Geometry check sheet. Reference: the model listing, model coordinates, mm. Face numbers are marked on the shaded views. A direction names the side the tool comes from. Give positions to 0.01 mm unless a question says otherwise; leave off trailing zeros. Write each loop counter-clockwise with the first axis right and the second up, starting at its lowest first coordinate (ties: lowest second). Pieces come first, ordered by that corner, then holes. Notation, with made-up numbers: (67.25, -17) - (96.25, -17) arc R8 ccw to (96.25, -10) - close; hole circle Ø10 at (40.5, 41.5). An arc over 180 degrees is marked (long way). Write item = value, one per line. Start each with the question number.
(1) Thickness scan on L1, parallel to Z at x = -8, y = 7.5; L2, parallel to X at y = 8, z = 2; L3, parallel to Z at x = -4.25, y = -2.25. Record the ranges inside material, lowest first.
(2) Depth check by flat-ended pin: pin 1 Ø1.8 at (y, z) = (8.96, 17.05) entering from +X; pin 2 Ø7 at (x, y) = (-0.5, 1.5) entering from -Z; pin 3 Ø1.5 at (x, z) = (5.5, 19) entering from +Y; pin 4 Ø3 at (y, z) = (8, 12.5) entering from -X. Enter the tip coordinate at first touch or a pass-through.
(3) Section check D-D, the plane y = -5.25. Enter the section's corners in (x, z).
(4) Section check A-A, the plane y = 2. Enter the section's corners in (x, z), plus the area to 3 significant figures.
(5) Draft check along Z on the marked faces 4, 5, 6 and 7. Enter one of: pulls with the +Z half, pulls with the -Z half, needs draft (parallel to the pull), parting line crosses it, or undercut.
(6) Access from +Z, -Z, +X, -X, +Y, -Y to the whole of each face (thin tool, end or side, straight path). Record for the marked faces 1, 2 and 3.
(7) Section check C-C, the plane z = 17.5. Enter the section's corners in (x, y).
(8) Section check B-B, the plane x = -1.75. Enter the section's corners in (y, z).
```python
from build123d import *

# Parameters (mm, degrees)
SKETCH_1_R           = 13
EXTRUDE_1_DEPTH      = 9
SKETCH_2_R           = 13
SKETCH_2_R_2         = 3.25
EXTRUDE_2_DEPTH      = 15
SKETCH_3_W           = 1.5
SKETCH_3_H           = 11.626426752
CUT_EXTRUDE_3_DEPTH  = 31.232432916
SKETCH_7_R           = 16.638234873
SKETCH_7_R_2         = 11
CUT_EXTRUDE_9_DEPTH  = 9
CUTOFF_START         = -3
SKETCH_8_W           = 6
SKETCH_8_H           = 5.368740975
SKETCH_8_H_2         = 7.372686293
CUTOFF_DEPTH         = 20
SKETCH_10_R          = 1.5
CUT_EXTRUDE_12_DEPTH = 32.638584039
CUT_EXTRUDE_START    = 3
SKETCH_9_W           = 5.7
SKETCH_9_H           = 7.372686293
SKETCH_9_H_2         = 5.368740975
CUT_EXTRUDE_11_DEPTH = 20


with BuildPart() as part:
    # Эскиз1 → Вытянуть1 (new body)
    with BuildSketch(Plane.XY):
        Circle(SKETCH_1_R)
        with BuildLine():
            Line((-4.5, 3.659234893), (-4.5, -3.659234893))
            ThreePointArc((-4.5, -3.659234893), (0, -5.8), (4.5, -3.659234893))
            Line((4.5, -3.659234893), (4.5, 3.659234893))
            ThreePointArc((4.5, 3.659234893), (0, 5.8), (-4.5, 3.659234893))
        make_face(mode=Mode.SUBTRACT)
    extrude(amount=EXTRUDE_1_DEPTH)

    # Эскиз2 → Вытянуть2 (add)
    with BuildSketch(Plane.XY.offset(9)):
        Circle(SKETCH_2_R)
        Circle(SKETCH_2_R_2, mode=Mode.SUBTRACT)
    extrude(amount=EXTRUDE_2_DEPTH)

    # Эскиз3 → Вытянуть3 (cut, through all)
    with BuildSketch(Plane(origin=(0, 0, 0), x_dir=(-1, 0, 0), z_dir=(0, 0, -1))):
        with Locations((0, 7.379803008)):
            Rectangle(SKETCH_3_W, SKETCH_3_H)
    extrude(amount=-CUT_EXTRUDE_3_DEPTH, mode=Mode.SUBTRACT)

    # Эскиз7 → Вытянуть9 (cut)
    with BuildSketch(Plane(origin=(0, 0, 0), x_dir=(-1, 0, 0), z_dir=(0, 0, -1))):
        Circle(SKETCH_7_R)
        Circle(SKETCH_7_R_2, mode=Mode.SUBTRACT)
    extrude(amount=-CUT_EXTRUDE_9_DEPTH, mode=Mode.SUBTRACT)

    # Эскиз8 → cutoff (cut)
    with BuildSketch(Plane(origin=(0, 0, 0), x_dir=(0, 0, -1), z_dir=(1, 0, 0)).offset(CUTOFF_START)):
        with Locations((-4.5, 8.290031546)):
            Rectangle(SKETCH_8_W, SKETCH_8_H)
        with Locations((-17, 9.292004205)):
            Rectangle(SKETCH_8_W, SKETCH_8_H_2)
    extrude(amount=-CUTOFF_DEPTH, mode=Mode.SUBTRACT)

    # Эскиз10 → Вытянуть12 (cut, through all)
    with BuildSketch(Plane.ZY.offset(3)):
        with Locations(Location((4.38073417, 8.174442111, 0), (0, 0, 90))):
            Circle(SKETCH_10_R)
        with Locations(Location((17.050484779, 8.958138025, 0), (0, 0, 90))):
            Circle(SKETCH_10_R)
    extrude(amount=-CUT_EXTRUDE_12_DEPTH, mode=Mode.SUBTRACT)

    # Эскиз9 → Вытянуть11 (cut)
    with BuildSketch(Plane(origin=(0, 0, 0), x_dir=(0, 0, -1), z_dir=(1, 0, 0)).offset(CUT_EXTRUDE_START)):
        with Locations((-17.050484779, 9.292004205)):
            Rectangle(SKETCH_9_W, SKETCH_9_H)
        with Locations((-4.38073417, 8.290031546)):
            Rectangle(SKETCH_9_W, SKETCH_9_H_2)
    extrude(amount=CUT_EXTRUDE_11_DEPTH, mode=Mode.SUBTRACT)


solid = part.part
```
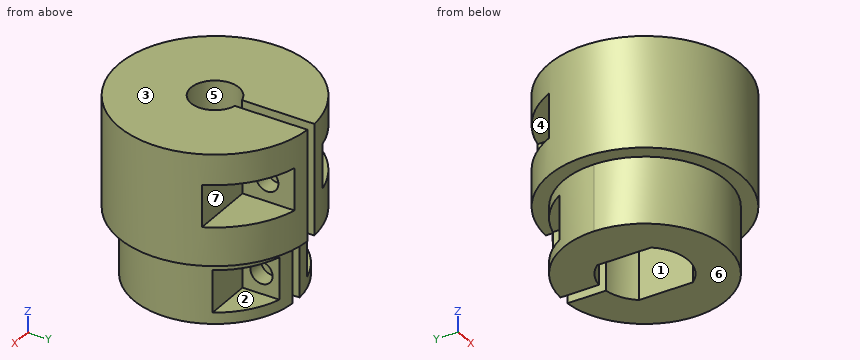
Model answer:
q1.L1 = 0 to 1.5, 7.5 to 14, 20 to 24
q1.L2 = -3 to -0.75, 0.75 to 3
q1.L3 = 9 to 24
q2.pin_1 = through
q2.pin_2 = 9
q2.pin_3 = 5.61
q2.pin_4 = -11.26
q3.outline = (-11.89, 9) - (-9.67, 9) - (-9.67, 0) - (-2.47, 0) - (-2.47, 9) - (2.47, 9) - (2.47, 0) - (9.67, 0) - (9.67, 9) - (11.89, 9) - (11.89, 24) - (-11.89, 24) - close
q4.outline = (-12.85, 9) - (-10.82, 9) - (-10.82, 0) - (-4.5, 0) - (-4.5, 9) - (-2.56, 9) - (-2.56, 24) - (-12.85, 24) - close; (2.56, 9) - (4.5, 9) - (4.5, 0) - (10.82, 0) - (10.82, 9) - (12.85, 9) - (12.85, 24) - (2.56, 24) - close
q4.area = 422 mm²
q5.face_4 = undercut
q5.face_5 = needs draft
q5.face_6 = pulls with the -Z half
q5.face_7 = undercut
q6.face_1 = -Z
q6.face_2 = +X, +Y
q6.face_3 = +Z, +X, -X, +Y, -Y
q7.outline = (-11.73, 5.61) arc R13 ccw (long way) to (11.73, 5.61) - (3, 5.61) - (3, 7.53) - (0.75, 7.53) - (0.75, 3.16) arc R3.25 cw (long way) to (-0.75, 3.16) - (-0.75, 7.53) - (-3, 7.53) - (-3, 5.61) - close; (-3, 10.39) - (-0.75, 10.39) - (-0.75, 12.98) arc R13 ccw to (-3, 12.65) - close; (0.75, 10.39) - (3, 10.39) - (3, 12.65) arc R13 ccw to (0.75, 12.98) - close
q8.outline = (-12.88, 9) - (-10.86, 9) - (-10.86, 0) - (-5.53, 0) - (-5.53, 9) - (-2.74, 9) - (-2.74, 24) - (-12.88, 24) - close; (2.74, 9) - (5.53, 9) - (5.53, 0) - (10.86, 0) - (10.86, 9) - (12.88, 9) - (12.88, 24) - (2.74, 24) - close; hole circle Ø3 at (8.17, 4.38); hole circle Ø3 at (8.96, 17.05)
